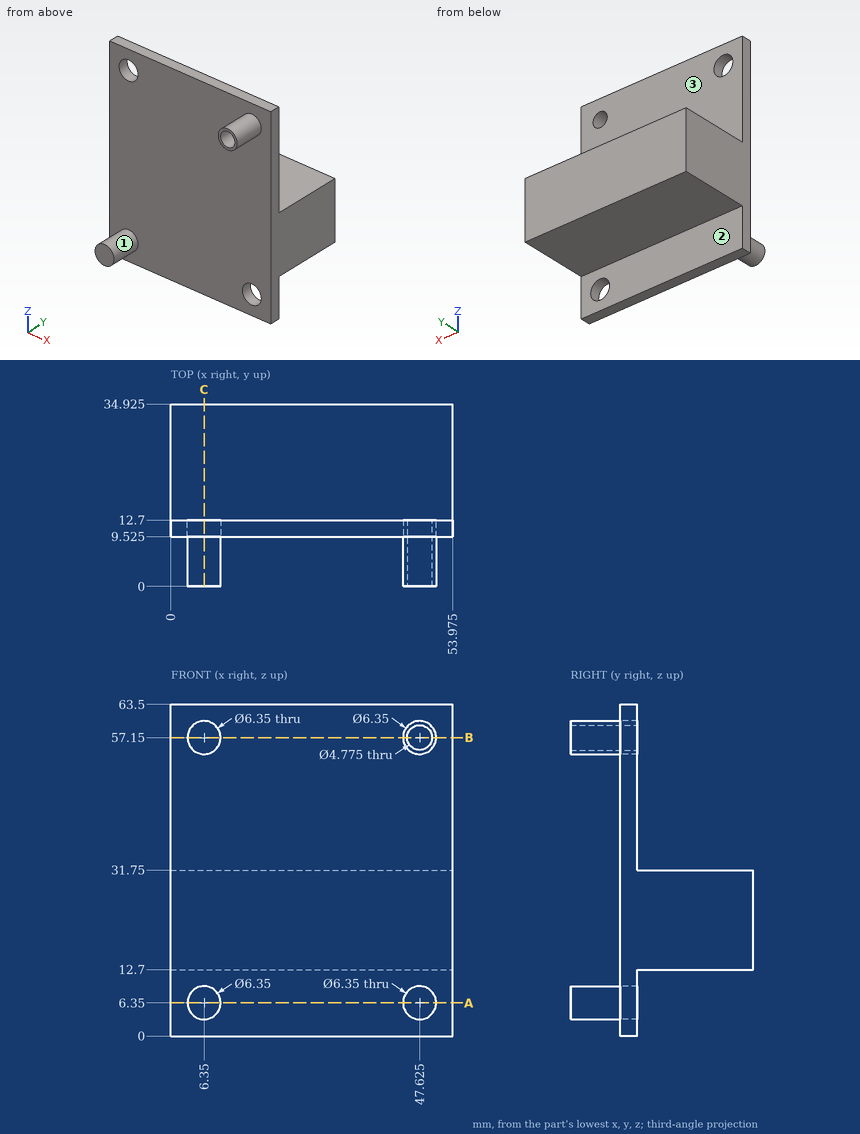
Design review of the part shown in the three views and the two pictorial views. Dimensions are in mm from the part's minimum x, y and z. A direction names the side the tool comes from. Give positions to 0.01 mm unless a question says otherwise; leave off trailing zeros. Order: outer loops, then holes, each group sorted by start corner. A loop starts at its lowest first (then second) coordinate and runs counter-clockwise, first axis right, second up. Notation, with made-up numbers: (1, -31) -> (30, -31) arc R38 cw to (30, 7) -> close; hole circle Ø5 at (34, 26). An arc over 180 degrees is marked (long way). Write each question's results on one line, items separated by ' | '. Start each with the question number.
Q1. For pin 1 (4 mm diameter, centred on y = 7, z = 47.5, fed in from +X); pin 2 (9.5 mm diameter, centred on x = 30, z = 52, fed in from +Y); pin 3 (4 mm diameter, centred on x = 6.5, z = 51.5, fed in from -Y) (3 decimals); pin 4 (18 mm diameter, centred on x = 21, y = 25.5, fed in from +Z), all flat-tipped, find the tip position at first contact; note any pin that passes through.
Q2. Add section A-A on z = 6.35. Give the boundary of the cut face in (x, y) (3 decimals).
Q3. Machinability: for the marked faces 1, 2 and 3, which of the approach directions +Z, -Z, +X, -X, +Y, -Y give a long, thin tool a straight path to every point of the face, cutting with its end or side? Answer none if there is none.
Q4. Add section B-B on z = 57.15. State how many separate pieces and enclosed holes the cut face has, and give its area (3 significant figures).
Q5. Wall thickness on L1, parallel to X at y = 10, z = 57 (1 decimal); L2, parallel to Z at x = 37, y = 26; L3, parallel to Y at x = 18, z = 6 (3 decimals): over which ranges is each line inside the solid? List them lowest first. Write a range as from..to.
Q6. Add section C-C on x = 6.35. Give the boundary of the cut face in (y, z) (3 decimals), and give its area (3 significant figures).
Found:
1) pin 1: passes through | pin 2: stops at y = 12.7 | pin 3: stops at y = 9.525 | pin 4: stops at z = 31.75
2) outline: (0, 9.525) -> (3.175, 9.525) -> (3.175, 0) -> (9.525, 0) -> (9.525, 9.525) -> (44.45, 9.525) -> (44.45, 12.7) -> (0, 12.7) -> close; (50.8, 9.525) -> (53.975, 9.525) -> (53.975, 12.7) -> (50.8, 12.7) -> close
3) face 1: -Y | face 2: -Z, +X, -X, +Y | face 3: +Z, +X, -X, +Y
4) separate pieces: 3 | enclosed holes: 0 | area: 151 mm2
5) L1: x = 0..3.2, 9.5..45.2, 50..54 | L2: z = 12.7..31.75 | L3: y = 9.525..12.7
6) outline: (0, 3.175) -> (9.525, 3.175) -> (9.525, 0) -> (12.7, 0) -> (12.7, 12.7) -> (34.925, 12.7) -> (34.925, 31.75) -> (12.7, 31.75) -> (12.7, 53.975) -> (9.525, 53.975) -> (9.525, 9.525) -> (0, 9.525) -> close; (9.525, 60.325) -> (12.7, 60.325) -> (12.7, 63.5) -> (9.525, 63.5) -> close | area: 665 mm2
